Verification items for the finished model (mm, model axes). A direction names the side the tool comes from. Round coordinates to 2 decimals unless told otherwise and drop trailing zeros. Loops run counter-clockwise (first coordinate to the right, second up) from the corner with the lowest first, then second, coordinate; pieces in that order, holes last. Notation, with made-up numbers: (45.5, 62.25) -> (76.5, 62.25) arc R26 cw to (76.5, 100.25) -> close; hole circle Ø8 at (15.5, -1). An arc over 180 degrees is marked (long way). Write item = value, one per line. Start each with the question number.
```python
from build123d import *

# Parameters (mm, degrees)
ENDCAP_1_DEPTH                  = 9.5
TAP_DRILL_FOR_M6X1_0_TAP1_D     = 6.5
TAP_DRILL_FOR_M6X1_0_TAP1_DEPTH = 12.5
TAP_DRILL_FOR_M6X1_0_TAP1_TIP   = 1.691842914
TAP_DRILL_FOR_M6X1_0_TAP2_D     = 6
SKETCH9_R                       = 3.65
CUT_EXTRUDE1_DEPTH              = 0.5


with BuildPart() as part:
    # Sketch3 → Endcap 1 (new body)
    with BuildSketch(Plane.XY):
        with BuildLine():
            Line((-21.7, 0), (-11.5, 0))
            Line((-11.5, 0), (-11.5, 0.6))
            Line((-11.5, 0.6), (-7.7, 4.4))
            Line((-7.7, 4.4), (-7.7, 7.78))
            Line((-7.7, 7.78), (-8.93, 9.01))
            ThreePointArc((-8.93, 9.01), (-9.658631808, 10.541368192), (-11.19, 11.27))
            Line((-11.19, 11.27), (-11.4, 11.48))
            Line((-11.4, 11.48), (-11.4, 13.51))
            Line((-11.4, 13.51), (-11.19, 13.719070796))
            ThreePointArc((-11.19, 13.719070796), (-9.661781613, 14.44408255), (-8.93, 15.969070796))
            Line((-8.93, 15.969070796), (-8.518177778, 16.379070796))
            Line((-8.518177778, 16.379070796), (8.518177778, 16.379070796))
            Line((8.518177778, 16.379070796), (8.93, 15.969070796))
            ThreePointArc((8.93, 15.969070796), (9.661781613, 14.44408255), (11.19, 13.719070796))
            Line((11.19, 13.719070796), (11.4, 13.51))
            Line((11.4, 13.51), (11.4, 11.48))
            Line((11.4, 11.48), (11.19, 11.27))
            ThreePointArc((11.19, 11.27), (9.658631808, 10.541368192), (8.93, 9.01))
            Line((8.93, 9.01), (7.7, 7.78))
            Line((7.7, 7.78), (7.7, 4.4))
            Line((7.7, 4.4), (11.5, 0.6))
            Line((11.5, 0.6), (11.5, 0))
            Line((11.5, 0), (21.7, 0))
            Line((21.7, 0), (23.2, 1.5))
            Line((23.2, 1.5), (23.2, 28))
            Line((23.2, 28), (21.7, 29.5))
            Line((21.7, 29.5), (5.8, 29.5))
            Line((5.8, 29.5), (5.05, 30.25))
            Line((5.05, 30.25), (-5.05, 30.25))
            Line((-5.05, 30.25), (-5.8, 29.5))
            Line((-5.8, 29.5), (-21.7, 29.5))
            Line((-21.7, 29.5), (-23.2, 28))
            Line((-23.2, 28), (-23.2, 1.5))
            Line((-23.2, 1.5), (-21.7, 0))
        make_face()
    extrude(amount=ENDCAP_1_DEPTH)

    # Tap Drill for M6x1.0 Tap1
    with Locations(Plane.XY.offset(9.5)):
        with Locations((-0.017990465, 24.379070796)):
            Hole(TAP_DRILL_FOR_M6X1_0_TAP1_D / 2, depth=TAP_DRILL_FOR_M6X1_0_TAP1_DEPTH)
            with Locations((0, 0, -(TAP_DRILL_FOR_M6X1_0_TAP1_DEPTH + TAP_DRILL_FOR_M6X1_0_TAP1_TIP / 2))):  # 125° drill point
                Cone(0, TAP_DRILL_FOR_M6X1_0_TAP1_D / 2, TAP_DRILL_FOR_M6X1_0_TAP1_TIP, mode=Mode.SUBTRACT)

    # Tap Drill for M6x1.0 Tap2 (through all)
    with Locations(Plane(origin=(23.2, 0, 0), x_dir=(0, 0, -1), z_dir=(1, 0, 0))):
        with Locations((-4.75, 25.5)):
            Hole(TAP_DRILL_FOR_M6X1_0_TAP2_D / 2)

    # Sketch9 → Cut-Extrude1 (cut)
    with BuildSketch(Plane(origin=(0, 30.25, 0), x_dir=(1, 0, 0), z_dir=(0, 1, 0))):
        with Locations((0, -5.399368506)):
            Circle(SKETCH9_R)
    extrude(amount=-CUT_EXTRUDE1_DEPTH, mode=Mode.SUBTRACT)


solid = part.part
```
(1) Section check C-C on x = 17. Enter the section's corners in (y, z), then the cut area to 3 significant figures.
(2) Access from +Z, -Z, +X, -X, +Y, -Y to the whole of each face (thin tool, end or side, straight path). Record for faces 1 (the cylindrical face through (3.48, 30, 4.3)), 2 (the cylindrical face through (9.68, 10.56, 4.68)), 3 (the flat face through (9.6, 2.5, 4.7)).
(3) Section check D-D on y = 25.5. Enter the section's corners in (x, z), then the cut area to 3 significant figures.
(4) Section check A-A on y = 3. Enter the section's corners in (x, z), then the cut area to 3 significant figures.
(5) Scan lines: line 1 (Y direction, x = 13, z = 4.75); line 2 (X direction, y = 12, z = 9); line 3 (Y direction, x = 0, z = 0.75). Record each from-to range of solid material in increasing order. Write a range as [from, to].
(6) Depth check by flat-ended pin: pin 1 Ø3 at (x, z) = (4, 4) entering from -Y; pin 2 Ø0.7 at (y, z) = (0.5, 5) entering from -X; pin 3 Ø3.5 at (x, z) = (0.5, 7) entering from +Y. Enter the tip coordinate at first touch or a pass-through.
(7) Draft check along X on faces 4 (the flat face through (0.1, 30.25, 1.5)), 5 (the flat face through (-11.4, 12, 5)), 6 (the flat face through (-22.5, 0.8, 4.7)). Enter one of: +X half, -X half, draft (parallel to the pull), parting line (faces both ways), or undercut.
(8) Section check B-B on x = 0. Enter the section's corners in (y, z).
Computed values:
q1.outline = (0, 0) -> (29.5, 0) -> (29.5, 9.5) -> (0, 9.5) -> close; hole circle Ø6 at (25.5, 4.75)
q1.area = 252 mm²
q2.face_1 = +Y
q2.face_2 = +Z, -Z
q2.face_3 = +Z, -Z, -Y
q3.outline = (-23.2, 0) -> (-3.07, 0) -> (-3.07, 1.75) -> (-23.2, 1.75) -> close; (-23.2, 7.75) -> (-3.07, 7.75) -> (-3.07, 9.5) -> (-23.2, 9.5) -> close; (3.03, 0) -> (23.2, 0) -> (23.2, 1.75) -> (3.03, 1.75) -> close; (3.03, 7.75) -> (23.2, 7.75) -> (23.2, 9.5) -> (3.03, 9.5) -> close
q3.area = 141 mm²
q4.outline = (-23.2, 0) -> (-9.1, 0) -> (-9.1, 9.5) -> (-23.2, 9.5) -> close; (9.1, 0) -> (23.2, 0) -> (23.2, 9.5) -> (9.1, 9.5) -> close
q4.area = 268 mm²
q5.line_1 = [0, 22.5], [28.5, 29.5]
q5.line_2 = [-23.2, -11.4], [11.4, 23.2]
q5.line_3 = [16.38, 21.13], [27.63, 30.25]
q6.pin_1 = 16.38
q6.pin_2 = -22.55
q6.pin_3 = 29.75
q7.face_4 = draft
q7.face_5 = undercut
q7.face_6 = -X half
q8.outline = (16.38, 0) -> (21.13, 0) -> (21.13, 9.5) -> (16.38, 9.5) -> close; (27.63, 0) -> (30.25, 0) -> (30.25, 1.75) -> (29.75, 1.75) -> (29.75, 9.05) -> (30.25, 9.05) -> (30.25, 9.5) -> (27.63, 9.5) -> (27.63, 6.86) arc R3 cw to (27.63, 2.64) -> close
